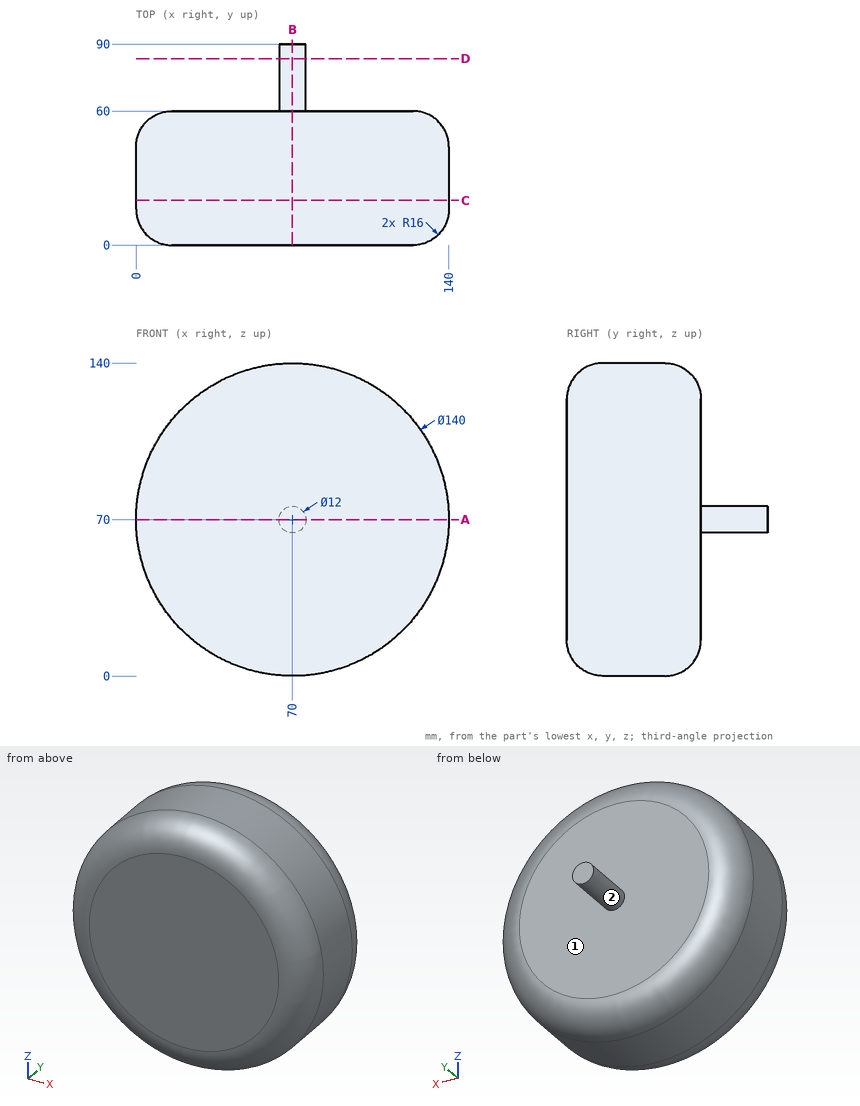
Check sheet for the drawn part. Datum: minimum x, y, z corner. Units: mm. Round coordinates to 2 decimals unless told otherwise and drop trailing zeros. Order: outer loops, then holes, each group sorted by start corner. A loop starts at its lowest first (then second) coordinate and runs counter-clockwise, first axis right, second up. Notation, with made-up numbers: (13, 89.5) - (44, 89.5) arc R31 ccw to (44, 113.5) - close; hole circle Ø10 at (-22, 58.5). An arc over 180 degrees is marked (long way). Use a Markdown table: item, result. Add a question column.
(1) Sectioned sample at D-D, the plane y = 83.5. Enter the section's corners in (x, z).
(2) Sectioned sample at A-A, the plane z = 70. Enter the section's corners in (x, y), and give its area (3 significant figures).
(3) Depth check by flat-ended pin: pin 1 (5 mm diameter, centred on x = 77, y = 78, fed in from +Z); pin 2 (4 mm diameter, centred on x = 16, y = 9, fed in from -Z); pin 3 (12 mm diameter, centred on x = 87, y = 74, fed in from +Z); pin 4 (1 mm diameter, centred on x = 22.5, z = 48, fed in from +Y). Enter the tip coordinate at first touch or a pass-through.
(4) Release check for a two-part mould opening along Z. For the marked faces 1 and 2 record: pulls with the +Z half, pulls with the -Z half, needs draft (parallel to the pull), parting line crosses it, or undercut.
(5) Sectioned sample at B-B, the plane x = 70. Enter the section's corners in (y, z).
(6) Sectioned sample at C-C, the plane y = 20. Enter the section's corners in (x, z), and give its area (3 significant figures).
(7) Material ranges on line 1 along Y through (x, z) = (82.5, 93); line 2 along Z through (x, y) = (128, 20.5); line 3 along Z through (x, y) = (70, 57), recorded low to high. Write a range as [from, to].
Answers below:
| question | item | result |
|---|---|---|
| 1 | outline | circle Ø12 at (70, 70) |
| 2 | outline | (0, 16) arc R16 ccw to (16, 0) - (124, 0) arc R16 ccw to (140, 16) - (140, 44) arc R16 ccw to (124, 60) - (76, 60) - (76, 90) - (64, 90) - (64, 60) - (16, 60) arc R16 ccw to (0, 44) - close |
| 2 | area | 8,540 mm² |
| 3 | pin 1 | z = 73.97 |
| 3 | pin 2 | z = 25.21 |
| 3 | pin 3 | through |
| 3 | pin 4 | y = 60 |
| 4 | face 1 | needs draft |
| 4 | face 2 | parting line crosses it |
| 5 | outline | (0, 16) arc R16 ccw to (16, 0) - (44, 0) arc R16 ccw to (60, 16) - (60, 64) - (90, 64) - (90, 76) - (60, 76) - (60, 124) arc R16 ccw to (44, 140) - (16, 140) arc R16 ccw to (0, 124) - close |
| 6 | outline | circle Ø140 at (70, 70) |
| 6 | area | 15,400 mm² |
| 7 | line 1 | [0, 60] |
| 7 | line 2 | [30.81, 109.19] |
| 7 | line 3 | [6.67, 133.33] |
